from build123d import *

# Parameters (mm, degrees)
SKETCH2_W           = 31.75
SKETCH2_H           = 31.75
SKETCH2_W_2         = 26.67
SKETCH2_H_2         = 26.67
BOSS_EXTRUDE1_DEPTH = 1174.75
CUT_EXTRUDE1_DEPTH  = 1176.286195199
SKETCH8_R           = 5.842


with BuildPart() as part:
    # Sketch2 → Boss-Extrude1 (new body)
    with BuildSketch(Plane(origin=(0, 0, 0), x_dir=(1, 0, 0), z_dir=(0, 1, 0))):
        Rectangle(SKETCH2_W, SKETCH2_H)
        Rectangle(SKETCH2_W_2, SKETCH2_H_2, mode=Mode.SUBTRACT)
    extrude(amount=BOSS_EXTRUDE1_DEPTH)

    # Sketch4 → Cut-Extrude1 (cut, through all)
    with BuildSketch(Plane.XY.offset(15.875)):
        Polygon((15.875, 0), (15.875, 37.838176565), (-15.875, 0), align=None)
        Polygon((15.875, 1174.75), (15.875, 1136.911823435), (-15.875, 1174.75), align=None)
    extrude(amount=-CUT_EXTRUDE1_DEPTH, mode=Mode.SUBTRACT)

    # Sweep2: sweep along a path in Sketch7
    with BuildLine(Plane(origin=(0, 0, 0), x_dir=(0, 0, -1), z_dir=(1, 0, 0))) as sweep2_path:
        ThreePointArc((-15.875, 608.965), (-37.465, 587.375), (-15.875, 565.785))
    # Sketch8 → Sweep2 (sweep)
    with BuildSketch(Plane.XY.offset(15.875)):
        with Locations((0, 608.965)):
            Circle(SKETCH8_R)
    sweep(path=sweep2_path.line)


solid = part.part
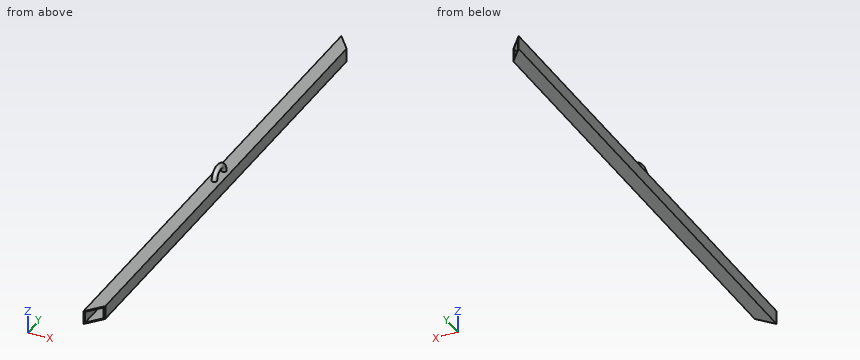
Verification items for the finished model (mm, model axes). Coordinates: 2 decimals unless noted, no trailing zeros. Order: outer loops, then holes, each group sorted by start corner. A loop starts at its lowest first (then second) coordinate and runs counter-clockwise, first axis right, second up.
1. Scan lines: line 1 (Z direction, x = -1, y = 658) (3 decimals); line 2 (Z direction, x = 1, y = 570) (3 decimals). Record each from-to range of solid material in increasing order.
Results found:
line 1: z = -15.875 to -13.335, 13.335 to 15.875
line 2: z = -15.875 to -13.335, 13.335 to 36.991
2. Go/stop test with flat-tipped pins: pin 1 Ø10 at (x, z) = (8, -0.5) entering from -Y; pin 2 Ø12 at (x, z) = (-4, 22) entering from +Y; pin 3 Ø6 at (x, y) = (4, 216) entering from +Z (3 decimals); pin 4 Ø12 at (x, z) = (-6, 16) entering from -Y. Record where each tip stops, or that it passes through.
Results found:
pin 1: passes through
pin 2: stops at y = 614.76
pin 3: stops at z = 15.875
pin 4: stops at y = 4.62
3. Sectioned sample at B-B, the plane y = 942.5. Record the cut outline in (x, z) (3 decimals).
Results found:
outline: (-15.875, -15.875) - (15.875, -15.875) - (15.875, 15.875) - (-15.875, 15.875) - close; hole (-13.335, -13.335) - (13.335, -13.335) - (13.335, 13.335) - (-13.335, 13.335) - close
4. Sectioned sample at A-A, the plane z = 1.5. Record the cut outline in (x, y) (3 decimals), and give its area (3 significant figures).
Results found:
outline: (-15.875, 0) - (-13.335, 3.027) - (-13.335, 1171.723) - (-15.875, 1174.75) - close; (13.335, 34.811) - (15.875, 37.838) - (15.875, 1136.912) - (13.335, 1139.939) - close
area: 5,780 mm2
